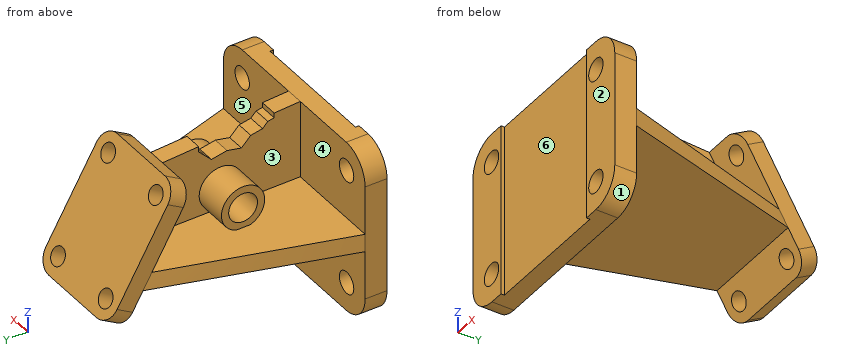
```python
from build123d import *

# Parameters (mm, degrees)
SKETCH2_R                = 4.826
BOSS_EXTRUDE1_DEPTH      = 9.652
CUT_EXTRUDE1_REACH       = 92.443
SKETCH4_W                = 57.404
SKETCH4_H                = 1.524
SKETCH7_R                = 3.937
BOSS_EXTRUDE2_DEPTH      = 7.874
RIB1_REACH               = 125.595
SKETCH11_WALL_W          = 310.061740512
SKETCH11_WALL_H          = 7.874
BOSS_EXTRUDE3_DEPTH      = 14.986
BOSS_EXTRUDE3_DEPTH_BACK = 20.066
SKETCH12_R               = 9.525
CUT_EXTRUDE2_DEPTH       = 126.168470882
CUT_EXTRUDE2_DEPTH_BACK  = 126.168470882
SKETCH12_3_R             = 6.35
CUT_EXTRUDE3_REACH       = 127.168


with BuildPart() as part:
    # Sketch2 → Boss-Extrude1 (new body)
    with BuildSketch(Plane(origin=(0, 0, 0), x_dir=(1, 0, 0), z_dir=(0, 1, 0))):
        with BuildLine():
            Line((35.052, -38.1), (-34.798, -38.1))
            ThreePointArc((-34.798, -38.1), (-43.778256121, -34.380256121), (-47.498, -25.4))
            Line((-47.498, -25.4), (-47.498, 25.4))
            ThreePointArc((-47.498, 25.4), (-43.778256121, 34.380256121), (-34.798, 38.1))
            Line((-34.798, 38.1), (35.052, 38.1))
            ThreePointArc((35.052, 38.1), (44.032256121, 34.380256121), (47.752, 25.4))
            Line((47.752, 25.4), (47.752, -25.4))
            ThreePointArc((47.752, -25.4), (44.032256121, -34.380256121), (35.052, -38.1))
        make_face()
        with Locations(Location((35.052, 25.4, 0), (0, 0, 270))):
            Circle(SKETCH2_R, mode=Mode.SUBTRACT)
        with Locations(Location((35.052, -25.4, 0), (0, 0, 90))):
            Circle(SKETCH2_R, mode=Mode.SUBTRACT)
        with Locations(Location((-35.052, -25.4, 0), (0, 0, 270))):
            Circle(SKETCH2_R, mode=Mode.SUBTRACT)
        with Locations(Location((-35.052, 25.4, 0), (0, 0, 90))):
            Circle(SKETCH2_R, mode=Mode.SUBTRACT)
    extrude(amount=BOSS_EXTRUDE1_DEPTH)

    # Sketch4 → Cut-Extrude1 (cut, up to next)
    with BuildSketch(Plane.XY.offset(38.1), mode=Mode.PRIVATE) as cut_extrude1_sk1:
        with Locations((0, 0.762)):
            Rectangle(SKETCH4_W, SKETCH4_H)
    cut_extrude1_tool1 = extrude(cut_extrude1_sk1.sketch, amount=-CUT_EXTRUDE1_REACH, mode=Mode.PRIVATE) & part.part
    add(cut_extrude1_tool1.solids().sort_by_distance((0, 0.762, 38.1))[0], mode=Mode.SUBTRACT)



with BuildPart() as body_2:
    # Sketch7 → Boss-Extrude2 (new body)
    with BuildSketch(Plane(origin=(0, 74.409783942, 42.960508789), x_dir=(0, 0.499999999999998, -0.8660254037844398), z_dir=(0, -0.8660254037844398, -0.499999999999998))):
        with BuildLine():
            Line((13.486432116, -23.876), (58.190432116, -23.876))
            ThreePointArc((58.190432116, -23.876), (63.758190911, -21.569758795), (66.064432116, -16.002))
            Line((66.064432116, -16.002), (66.064432116, 16.002))
            ThreePointArc((66.064432116, 16.002), (63.758190911, 21.569758795), (58.190432116, 23.876))
            Line((58.190432116, 23.876), (13.486432116, 23.876))
            ThreePointArc((13.486432116, 23.876), (7.918673321, 21.569758795), (5.612432116, 16.002))
            Line((5.612432116, 16.002), (5.612432116, -16.002))
            ThreePointArc((5.612432116, -16.002), (7.918673321, -21.569758795), (13.486432116, -23.876))
        make_face()
        with Locations((13.740432116, 16.002)):
            Circle(SKETCH7_R, mode=Mode.SUBTRACT)
        with Locations(Location((13.740432116, -16.002, 0), (0, 0, 180))):
            Circle(SKETCH7_R, mode=Mode.SUBTRACT)
        with Locations((57.936432116, -16.002)):
            Circle(SKETCH7_R, mode=Mode.SUBTRACT)
        with Locations(Location((57.936432116, 16.002, 0), (0, 0, 180))):
            Circle(SKETCH7_R, mode=Mode.SUBTRACT)
    extrude(amount=BOSS_EXTRUDE2_DEPTH)


with BuildPart() as part_1:
    add(part.part)

    add(body_2.part)  # Loft1 merges body 2
    # Sketch10 → Loft1 section 0
    with BuildSketch(Plane(origin=(0, 67.590699913, 39.023508789), x_dir=(1, 0, 0), z_dir=(0, -0.8660254037844398, -0.49999999999999806))):
        with BuildLine():
            Line((23.876, -48.986339597), (-23.876, -48.986339597))
            Line((-23.876, -48.986339597), (-23.876, -41.13459362))
            Line((-23.876, -41.13459362), (23.876, -41.13459362))
            Line((23.876, -41.13459362), (23.876, -48.986339597))
        make_face()
    # Sketch8 → Loft1 section 1
    with BuildSketch(Plane(origin=(0, 9.652, 0), x_dir=(1, 0, 0), z_dir=(0, 1, 0))):
        with BuildLine():
            Line((47.752, -3.937), (-47.498, -3.937))
            Line((-47.498, -3.937), (-47.498, 3.937))
            Line((-47.498, 3.937), (47.752, 3.937))
            Line((47.752, 3.937), (47.752, -3.937))
        make_face()
    loft()

    # Sketch11 wall → Rib1 (add, up to next)
    with BuildSketch(Plane(origin=(0, 40.024457985, 36.1315), x_dir=(0, 0.997906295589, -0.064676311144), z_dir=(0, 0.064676311144, 0.997906295589)), mode=Mode.PRIVATE) as rib1_sk1:
        Rectangle(SKETCH11_WALL_W, SKETCH11_WALL_H)
    rib1_tool1 = extrude(rib1_sk1.sketch, amount=-RIB1_REACH, mode=Mode.PRIVATE) - part_1.part
    add(rib1_tool1.solids().sort_by_distance((0, 40.024457985, 36.1315))[0])

    # Sketch12 → Boss-Extrude3 (add, two sides: drawn at the far end of the back side and taken through both)
    with BuildSketch(Plane.ZY.offset(3.937).offset(-BOSS_EXTRUDE3_DEPTH_BACK)):
        with Locations((12.7, 44.704)):
            Circle(SKETCH12_R)
    extrude(amount=BOSS_EXTRUDE3_DEPTH + BOSS_EXTRUDE3_DEPTH_BACK)

    # Sketch12_3 → Cut-Extrude2 (cut, two sides: drawn at the far end of the back side and taken through both)
    with BuildSketch(Plane.ZY.offset(3.937).offset(-CUT_EXTRUDE2_DEPTH_BACK)):
        with Locations((12.7, 44.704)):
            Circle(SKETCH12_3_R)
    extrude(amount=CUT_EXTRUDE2_DEPTH + CUT_EXTRUDE2_DEPTH_BACK, mode=Mode.SUBTRACT)

    # Sketch13 → Cut-Extrude3 (cut, up to next)
    with BuildSketch(Plane.ZY.offset(3.937), mode=Mode.PRIVATE) as cut_extrude3_sk1:
        Polygon((32.789961939, 54.446931247), (29.83831511, 51.495284418), (27.177726093, 48.8346954), (28.508020602, 41.928118952), (27.177726093, 35.60023156), (31.314138525, 31.463819128), (32.308134502, 26.303225622), (34.659879511, 23.951480612), (35.196750543, 21.164172387), (41.131268047, 21.164172387), (39.117849331, 54.446931247), align=None)
    cut_extrude3_tool1 = extrude(cut_extrude3_sk1.sketch, amount=-CUT_EXTRUDE3_REACH, mode=Mode.PRIVATE) & part_1.part
    add(cut_extrude3_tool1.solids().sort_by_distance((-3.937, 38.754988, 34.773506))[0], mode=Mode.SUBTRACT)


solid = part_1.part
```
Here's how the part is built. I have some questions about the finished solid (model axes, mm). Face numbers are marked on the shaded views. A direction names the side the tool comes from. Give positions to 0.01 mm unless a question says otherwise; leave off trailing zeros. Order: outer loops, then holes, each group sorted by start corner. A loop starts at its lowest first (then second) coordinate and runs counter-clockwise, first axis right, second up. Notation, with made-up numbers: M -7.5,4.5 L 43.5,4.5 A18 cw 43.5,16.5 Z; hole C -7,0.25 d7. An arc over 180 degrees is marked long. Use a Markdown table: item, result. Add a question column.
1. On a 3-axis mill with a long thin cutter (end or side, diameter ignored), from which of +Z, -Z, +X, -X, +Y, -Y can I reach the whole of each face in a straight line? I mean the marked faces 4, 5 and 6. Say none if no direction works.
2. If we mould it in two halves opening along Y, with no side actions, what happens to the marked faces 1, 2 and 3? For each: +Y half, -Y half, draft (parallel to the pull), parting line (faces both ways), or undercut.
3. Suppose I cut it at B-B (x = -32). Give the number of separate pieces and of enclosed holes in the cut face, and give its area (3 significant figures).
4. For pin 1 Ø1.7 at (x, z) = (-1, 36.5) entering from +Y; pin 2 Ø8 at (y, z) = (60.5, 7) entering from -X; pin 3 Ø7.5 at (x, z) = (-35.052, -25.4) entering from -Y; pin 4 Ø15 at (y, z) = (40, 11.5) entering from +X, each with a flat end and sliding along its axis, tell me the tip position at first contact or that it passes through.
5. Suppose I cut it at A-A (z = 12.7). List the corners of the cut face in (x, y) for me, and give its area (3 significant figures).
6. I need wall thicknesses on probe 1 along X at (y, z) = (4, 25); probe 2 along Y at (x, z) = (-39, 31.5); probe 3 along Z at (x, y) = (28, 12). Which ranges of each line are inside material? Lowest first, please. Write a range as from..to.
Results list:
| question | item | result |
|---|---|---|
| 1 | face 4 | +Z, -X |
| 1 | face 5 | +Z, +X |
| 1 | face 6 | +Z, -Z, -Y |
| 2 | face 1 | draft |
| 2 | face 2 | -Y half |
| 2 | face 3 | undercut |
| 3 | separate pieces | 3 |
| 3 | enclosed holes | 0 |
| 3 | area | 988 mm² |
| 4 | pin 1 | stops at y = 78.63 |
| 4 | pin 2 | stops at x = -32.83 |
| 4 | pin 3 | passes through |
| 4 | pin 4 | stops at x = 16.13 |
| 5 | outline | M -47.5,0 L -28.7,0 L -28.7,1.52 L 28.7,1.52 L 28.7,0 L 47.75,0 L 47.75,9.65 L 3.94,9.65 L 3.94,35.18 L 16.13,35.18 L 16.13,38.35 L -18.92,38.35 L -18.92,35.18 L -3.94,35.18 L -3.94,9.65 L -47.5,9.65 Z; M -23.88,82.79 L -3.94,82.79 L -3.94,54.23 L -18.92,54.23 L -18.92,51.05 L 16.13,51.05 L 16.13,54.23 L 3.94,54.23 L 3.94,82.79 L 23.88,82.79 L 23.88,91.88 L -23.88,91.88 Z |
| 5 | area | 1,910 mm² |
| 6 | probe 1 | x = -47.5..-39.86, -30.24..30.24, 39.86..47.75 |
| 6 | probe 2 | y = 0..9.65 |
| 6 | probe 3 | z = -3.92..3.92 |
